The model under review builds one solid part; all positions refer to its coordinate system, in mm. Face numbers are marked on the shaded views. A direction names the side the tool comes from. Round coordinates to 2 decimals unless told otherwise and drop trailing zeros. Order: outer loops, then holes, each group sorted by start corner. A loop starts at its lowest first (then second) coordinate and runs counter-clockwise, first axis right, second up. Notation, with made-up numbers: M 62.25,21.25 L 72.25,21.25 A12 cw 72.25,40.25 Z; hole C 49,-7 d2. An arc over 180 degrees is marked long. Answer as a JSON object with one key per item and string values. Group by question number.
1) Consider section C-C, the plane x = -10.5. Write out the cut boundary in (y, z), then the cut area to 3 significant figures.
2) Consider section A-A, the plane z = -2. Write out the cut boundary in (x, y), then the cut area to 3 significant figures.
3) Consider section B-B, the plane y = -7. Write out the cut boundary in (x, z).
4) To check wall thickness, follow line 1 (Z direction, x = 46, y = -5); line 2 (Y direction, x = -7.5, z = -13.5); line 3 (X direction, y = -4, z = -11). State the ranges of each line that lie inside material, in increasing order.
5) Insertion check: pin 1 Ø1 at (y, z) = (25.5, -21.5) entering from +X; pin 2 Ø4 at (x, y) = (-25.5, 0.5) entering from -Z; pin 3 Ø6.5 at (y, z) = (-1.5, -18) entering from +X. Each pin has a flat end and moves straight along its axis. Give the tip position at first contact, or say it passes through.
6) For the marked faces 1, 2 and 3, list the 3-axis set-ups (+Z, -Z, +X, -X, +Y, -Y) from which the entire face can be reached by the end or side of a thin tool; tool diameter is ignored.
7) The part is to be moulded in two halves that separate along X. For the marked faces 4, 5 and 6, say which applies: +X half, -X half, draft (parallel to the pull), parting line (faces both ways), or undercut.
8) Consider section D-D, the plane x = -25. Write out the cut boundary in (y, z), then the cut area to 3 significant figures.
```python
from build123d import *

# Parameters (mm, degrees)
F1_DEPTH = 12.7
F3_DEPTH = 12.7
F4_R     = 6.35
F5_DEPTH = 12.7
F7_DEPTH = 2.54
F7_TAPER = 45


with BuildPart() as f1:
    # F0 (on Top) → F1 (new body)
    with BuildSketch(Plane.XY):
        Polygon((-40.7569743693, 40.2890797282), (-40.7569743693, -10.5109202718), (48.1430256307, -10.5109202718), (48.1430256307, 2.1890797282), (60.8430256307, 2.1890797282), (60.8430256307, 14.8890797282), (10.0430256307, 40.2890797282), align=None)
    extrude(amount=F1_DEPTH)

    # F2 (on face) → F3 (join)
    with BuildSketch(Plane.XY.offset(12.7)):
        Polygon((-40.7569743693, 40.2890797282), (-40.7569743693, -10.5109202718), (-15.3569743693, -10.5109202718), (-15.3569743693, 2.1890797282), (48.1430256307, 2.1890797282), (60.8430256307, 2.1890797282), (60.8430256307, 14.8890797282), (10.0430256307, 40.2890797282), align=None)
    extrude(amount=F3_DEPTH)

    # F4 (on face) → F5 (cut)
    with BuildSketch(Plane.XY.offset(25.4)):
        with Locations((-28.0569743693, 2.1890797282)):
            Circle(F4_R)
    extrude(amount=-F5_DEPTH, mode=Mode.SUBTRACT)

    # F6 (on face) → F7 (cut)
    with BuildSketch(Plane.XY.offset(25.4)):
        Polygon((22.7430256307, 14.8890797282), (35.4430256307, 14.8890797282), (35.4430256307, 27.5890797282), (22.7430256307, 33.9390797282), align=None)
    extrude(amount=-F7_DEPTH, taper=F7_TAPER, mode=Mode.SUBTRACT)


with BuildPart() as f8_1:
    # F8: instance of F1
    add(f1.part.mirror(Plane(origin=(3.3794453838, 13.0859933084, 0), x_dir=(1, 0, 0), z_dir=(0, 0, -1))))


solid = f8_1.part
```
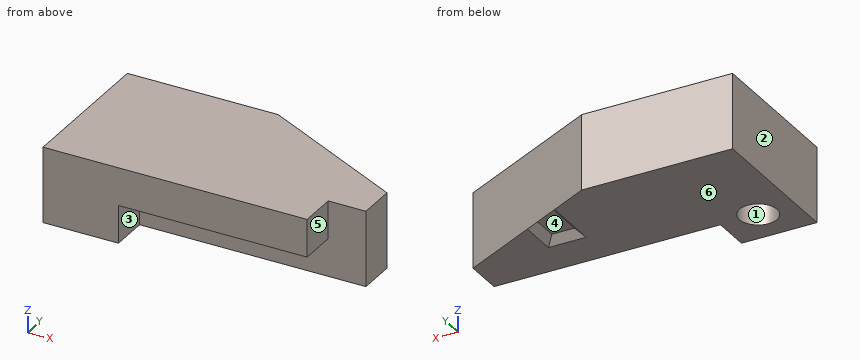
Results list:
{
 "1": {"outline": "M -10.51,-12.7 L 2.19,-12.7 L 2.19,-25.4 L 40.29,-25.4 L 40.29,0 L -10.51,0 Z", "area": "1,130 mm^2"},
 "2": {"outline": "M -40.76,-10.51 L 48.14,-10.51 L 48.14,2.19 L 60.84,2.19 L 60.84,14.89 L 10.04,40.29 L -40.76,40.29 Z", "area": "4,350 mm^2"},
 "3": {"outline": "M -40.76,-25.4 L -15.36,-25.4 L -15.36,-12.7 L 48.14,-12.7 L 48.14,0 L -40.76,0 Z"},
 "4": {"line 1": "-12.7 to 0", "line 2": "2.19 to 40.29", "line 3": "-40.76 to 48.14"},
 "5": {"pin 1": "x = 40.62", "pin 2": "z = -12.7", "pin 3": "x = -15.36"},
 "6": {"face 1": "-Z", "face 2": "+Z, -Z, -X, +Y, -Y", "face 3": "-Z, +X, -Y"},
 "7": {"face 4": "undercut", "face 5": "+X half", "face 6": "draft"},
 "8": {"outline": "M -10.51,-25.4 L -3.38,-25.4 L -3.38,-12.7 L 7.75,-12.7 L 7.75,-25.4 L 40.29,-25.4 L 40.29,0 L -10.51,0 Z", "area": "1,150 mm^2"}
}
